from build123d import *

# Parameters (mm, degrees)
SKETCH_1_W               = 100
SKETCH_1_H               = 80
EXTRUDE_1_DEPTH          = 5
SKETCH_2_R               = 1.5
CUT_EXTRUDE_1_DEPTH      = 6
MIRROR_2_COPY_1_SKETCH_R = 1.5
MIRROR_2_COPY_1_DEPTH    = 6
SKETCH_4_W               = 100
SKETCH_4_H               = 20
EXTRUDE_2_DEPTH          = 3
SKETCH_5_W               = 83
SKETCH_5_H               = 20
EXTRUDE_3_DEPTH          = 3
SKETCH_6_W               = 106
SKETCH_6_H               = 20
EXTRUDE_4_DEPTH          = 3
SKETCH_7_R               = 1.25
CUT_EXTRUDE_2_DEPTH      = 6
CUT_EXTRUDE_3_DEPTH      = 2
SKETCH_9_W               = 15
SKETCH_9_H               = 10
CUT_EXTRUDE_4_DEPTH      = 6


with BuildPart() as part:
    # 草图1 → 凸台-拉伸1 (new body)
    with BuildSketch(Plane(origin=(0, 0, 0), x_dir=(1, 0, 0), z_dir=(0, 1, 0))):
        Rectangle(SKETCH_1_W, SKETCH_1_H)
    extrude(amount=EXTRUDE_1_DEPTH)

    # 草图2 → 切除-拉伸1 (cut, through all)
    with BuildSketch(Plane(origin=(0, 5, 0), x_dir=(1, 0, 0), z_dir=(0, 1, 0))):
        with Locations((20, 30)):
            Circle(SKETCH_2_R)
    cut_extrude_1 = extrude(amount=-CUT_EXTRUDE_1_DEPTH, mode=Mode.SUBTRACT)

    # 镜向1: 切除-拉伸1 across plane
    add(cut_extrude_1.mirror(Plane.ZY), mode=Mode.SUBTRACT)

    # 镜向2: 切除-拉伸1 across plane
    add(cut_extrude_1.mirror(Plane.XY), mode=Mode.SUBTRACT)

    # 镜向2 copy 1 sketch → 镜向2 copy 1 (cut, through all)
    with BuildSketch(Plane(origin=(0, 5, 0), x_dir=(-1, 0, 0), z_dir=(0, 1, 0))):
        with Locations((20, 30)):
            Circle(MIRROR_2_COPY_1_SKETCH_R)
    extrude(amount=-MIRROR_2_COPY_1_DEPTH, mode=Mode.SUBTRACT)

    # 草图4 → 凸台-拉伸2 (add)
    with BuildSketch(Plane.XY.offset(40)):
        with Locations((0, 10)):
            Rectangle(SKETCH_4_W, SKETCH_4_H)
    extrude(amount=EXTRUDE_2_DEPTH)

    # 草图5 → 凸台-拉伸3 (add)
    with BuildSketch(Plane.ZY.offset(50)):
        with Locations((1.5, 10)):
            Rectangle(SKETCH_5_W, SKETCH_5_H)
    extrude_3 = extrude(amount=EXTRUDE_3_DEPTH)

    # 镜向3: 凸台-拉伸3 across plane
    add(extrude_3.mirror(Plane.ZY))

    # 草图6 → 凸台-拉伸4 (add)
    with BuildSketch(Plane(origin=(0, 0, -40), x_dir=(-1, 0, 0), z_dir=(0, 0, -1))):
        with Locations((0, 10)):
            Rectangle(SKETCH_6_W, SKETCH_6_H)
    extrude(amount=EXTRUDE_4_DEPTH)

    # 草图7 → 切除-拉伸2 (cut, through all)
    with BuildSketch(Plane(origin=(0, 5, 0), x_dir=(1, 0, 0), z_dir=(0, 1, 0))):
        with Locations((5.45, 20.04)):
            Circle(SKETCH_7_R)
        with Locations((-30.55, 20.04)):
            Circle(SKETCH_7_R)
        with Locations((-30.55, -15.96)):
            Circle(SKETCH_7_R)
        with Locations((5.45, -15.96)):
            Circle(SKETCH_7_R)
    extrude(amount=-CUT_EXTRUDE_2_DEPTH, mode=Mode.SUBTRACT)

    # 草图8 → 切除-拉伸3 (cut)
    with BuildSketch(Plane.XZ):
        Polygon((-28.01123046, 17.425759277), (-30.55, 18.891518554), (-33.08876954, 17.425759277), (-33.08876954, 14.494240723), (-30.55, 13.028481446), (-28.01123046, 14.494240723), align=None)
        Polygon((-30.55, -17.0377786), (-33.15, -18.5388893), (-33.15, -21.5411107), (-30.55, -23.0422214), (-27.95, -21.5411107), (-27.95, -18.5388893), align=None)
        Polygon((5.45, 18.9622214), (2.85, 17.4611107), (2.85, 14.4588893), (5.45, 12.9577786), (8.05, 14.4588893), (8.05, 17.4611107), align=None)
        Polygon((5.45, -17.0377786), (2.85, -18.5388893), (2.85, -21.5411107), (5.45, -23.0422214), (8.05, -21.5411107), (8.05, -18.5388893), align=None)
    extrude(amount=-CUT_EXTRUDE_3_DEPTH, mode=Mode.SUBTRACT)

    # 草图9 → 切除-拉伸4 (cut, through all)
    with BuildSketch(Plane(origin=(0, 5, 0), x_dir=(1, 0, 0), z_dir=(0, 1, 0))):
        with Locations((40, 15)):
            Rectangle(SKETCH_9_W, SKETCH_9_H)
    extrude(amount=-CUT_EXTRUDE_4_DEPTH, mode=Mode.SUBTRACT)


solid = part.part
Geometry: final body of the model. Coordinates: model frame, mm. A direction names the side the tool comes from. Coordinates: 2 decimals unless noted, no trailing zeros. Order: outer loops, then holes, each group sorted by start corner. A loop starts at its lowest first (then second) coordinate and runs counter-clockwise, first axis right, second up. Notation, with made-up numbers: (26.5, 20.25) - (74.5, 20.25) arc R22 cw to (74.5, 59.25) - close; hole circle Ø9 at (54.25, -32). An arc over 180 degrees is marked (long way). Use one line per item in the form item = value.
1) Section D-D (x = 20). Return loops of the section in (y, z), then the cut area to 3 significant figures.
Solutions:
outline = (0, -43) - (20, -43) - (20, -40) - (5, -40) - (5, -31.5) - (0, -31.5) - close; (0, -28.5) - (5, -28.5) - (5, 28.5) - (0, 28.5) - close; (0, 31.5) - (5, 31.5) - (5, 40) - (20, 40) - (20, 43) - (0, 43) - close
area = 490 mm^2
2) Set-up query: faces 4 (the face through (1, 0, 1)), 5 (the face through (40, 3, -10)), 6 (the face through (-50, 13, -1)), 7 (the face through (4, 2, -21)). Return all of +Z, -Z, +X, -X, +Y, -Y with unobstructed straight access to the full face (end or side cutting, diameter ignored); none if empty.
Solutions:
face_4 = +Z, -Z, +X, -X, -Y
face_5 = +Y, -Y
face_6 = +Y
face_7 = -Y
3) Section A-A (x = 40). Return loops of the section in (y, z).
Solutions:
outline = (0, -43) - (20, -43) - (20, -40) - (5, -40) - (5, -20) - (0, -20) - close; (0, -10) - (5, -10) - (5, 40) - (20, 40) - (20, 43) - (0, 43) - close
4) Pin query (flat end, axial travel): pin 1 (5 mm diameter, centred on x = -30, z = 0.5, fed in from +Y); pin 2 (2.5 mm diameter, centred on x = 4.5, z = 16, fed in from -Y); pin 3 (2 mm diameter, centred on x = 5.45, z = -20.04, fed in from +Y). Return the tip coordinate at first contact, or that it passes through.
Solutions:
pin_1 = 5
pin_2 = 2
pin_3 = through
5) Section C-C (y = 11). Return loops of the section in (x, z).
Solutions:
outline = (-53, -43) - (53, -43) - (53, 43) - (-53, 43) - close; hole (-50, -40) - (50, -40) - (50, 40) - (-50, 40) - close
6) Section B-B (z = 30). Return loops of the section in (x, y).
Solutions:
outline = (-53, 0) - (-21.5, 0) - (-21.5, 5) - (-50, 5) - (-50, 20) - (-53, 20) - close; (-18.5, 0) - (18.5, 0) - (18.5, 5) - (-18.5, 5) - close; (21.5, 0) - (53, 0) - (53, 20) - (50, 20) - (50, 5) - (21.5, 5) - close
7) Ray query, L1, parallel to Z at x = -20, y = 1.9; L2, parallel to Z at x = -30.55, y = 4.1; L3, parallel to X at y = 2.15, z = -30. Return the intervals inside material, ascending.
Solutions:
L1 = -43 to -31.5, -28.5 to 28.5, 31.5 to 43
L2 = -43 to -21.29, -18.79 to 14.71, 17.21 to 43
L3 = -53 to -21.5, -18.5 to 18.5, 21.5 to 53
8) Mould query, pull axis Z, two halves, no side actions, for faces 1 (the face through (5.18, 3.52, 17.18)), 2 (the face through (1, 10, -43)), 3 (the face through (53, 10, 1)). Classes: +Z half, -Z half, draft (parallel to the pull), parting line (faces both ways), or undercut.
Solutions:
face_1 = undercut
face_2 = -Z half
face_3 = draft
